CAD build for the part. Positions are in the model's coordinates, mm. A direction names the side the tool comes from. Round coordinates to 2 decimals unless told otherwise and drop trailing zeros. Loops run counter-clockwise (first coordinate to the right, second up) from the corner with the lowest first, then second, coordinate; pieces in that order, holes last. Notation, with made-up numbers: M 42.25,-19.75 L 82.25,-19.75 A25 cw 82.25,7.25 Z; hole C 34,34.5 d9. An arc over 180 degrees is marked long. Use a Markdown table: item, result. Add a question column.
(1) Band-saw the part on B-B, the plane x = 22.5. Write the cut outline in (y, z) (3 decimals), and give its area (3 significant figures).
(2) Which spindle directions (+Z, -Z, +X, -X, +Y, -Y) get a long thin tool onto all of the face, cutting with end or side? Do faces 1 (the face through (40, 2, -20.4)), 2 (the face through (23.425, 2, -35)), 3 (the face through (4, 2, -20.4)). Say none if no direction does.
(3) Band-saw the part on C-C, the plane y = 1.5. Give the number of separate pieces and of enclosed holes in the cut face, and give its area (3 significant figures).
(4) Wall check: L1, parallel to X at y = 0.65, z = -18 (3 decimals); L2, parallel to Z at x = 5, y = 2.65; L3, parallel to Z at x = 22, y = 2.8. Give the ranges that are in metal, low to high.
(5) Two-plate mould, pull along X, no slides. Class faces 4 (the face through (0, 1, -37)), 5 (the face through (30, 2, -48)), 6 (the face through (40, 1, 0)): released by +X, released by -X, zero draft, split by the parting line, or undercut.
(6) Band-saw the part on A-A, the plane x = 41. Write the cut outline in (y, z), and give its area (3 significant figures).
(7) Flat gauge pins, fed straight in: P1, Ø5, axis at x = 20, z = -11.5, coming from the -Y side; P2, Ø1.5, axis at x = 20, y = 1, coming from the -Z side. Where does each tip first touch, or does it go through?
from build123d import *

# Parameters (mm, degrees)
SKETCH1_W           = 45
SKETCH1_H           = 50
BOSS_EXTRUDE1_DEPTH = 3
SKETCH2_W           = 20
SKETCH2_H           = 3
SKETCH2_W_2         = 22
SKETCH2_W_3         = 7.5
SKETCH2_W_4         = 9
CUT_EXTRUDE1_DEPTH  = 4
SKETCH4_W           = 7.5
SKETCH4_H           = 0.1
SKETCH4_W_2         = 9
CUT_EXTRUDE2_DEPTH  = 4


with BuildPart() as part:
    # Sketch1 → Boss-Extrude1 (new body)
    with BuildSketch(Plane(origin=(0, 0, 0), x_dir=(1, 0, 0), z_dir=(0, 1, 0))):
        with Locations((22.5, 25)):
            Rectangle(SKETCH1_W, SKETCH1_H)
    extrude(amount=BOSS_EXTRUDE1_DEPTH)

    # Sketch2 → Cut-Extrude1 (cut, through all)
    with BuildSketch(Plane(origin=(0, 3, 0), x_dir=(1, 0, 0), z_dir=(0, 1, 0))):
        with Locations((20, 48.5)):
            Rectangle(SKETCH2_W, SKETCH2_H)
        with Locations((24, 1.5)):
            Rectangle(SKETCH2_W_2, SKETCH2_H)
        with Locations((3.75, 22)):
            Rectangle(SKETCH2_W_3, SKETCH2_H)
        with Locations((40.5, 22)):
            Rectangle(SKETCH2_W_4, SKETCH2_H)
        Polygon((21.050252532, 21.5), (23.949747468, 21.5), (26, 23.550252532), (26, 26.449747468), (23.949747468, 28.5), (21.050252532, 28.5), (19, 26.449747468), (19, 23.550252532), align=None)
        with BuildLine():
            Line((21.575, 31.5), (21.575, 38.25))
            ThreePointArc((21.575, 38.25), (22.5, 39.175), (23.425, 38.25))
            Line((23.425, 38.25), (23.425, 31.5))
            ThreePointArc((23.425, 31.5), (22.5, 30.575), (21.575, 31.5))
        make_face()
        with BuildLine():
            Line((23.425, 18.5), (23.425, 11.75))
            ThreePointArc((23.425, 11.75), (22.5, 10.825), (21.575, 11.75))
            Line((21.575, 11.75), (21.575, 18.5))
            ThreePointArc((21.575, 18.5), (22.5, 19.425), (23.425, 18.5))
        make_face()
    extrude(amount=-CUT_EXTRUDE1_DEPTH, mode=Mode.SUBTRACT)

    # Sketch4 → Cut-Extrude2 (cut, through all)
    with BuildSketch(Plane(origin=(0, 3, 0), x_dir=(1, 0, 0), z_dir=(0, 1, 0))):
        with Locations((3.75, 23.55)):
            Rectangle(SKETCH4_W, SKETCH4_H)
        with Locations((3.75, 20.45)):
            Rectangle(SKETCH4_W, SKETCH4_H)
        with Locations((40.5, 20.45)):
            Rectangle(SKETCH4_W_2, SKETCH4_H)
        with Locations((40.5, 23.55)):
            Rectangle(SKETCH4_W_2, SKETCH4_H)
    extrude(amount=-CUT_EXTRUDE2_DEPTH, mode=Mode.SUBTRACT)


solid = part.part
Return value:
| question | item | result |
|---|---|---|
| 1 | outline | M 0,-47 L 3,-47 L 3,-39.175 L 0,-39.175 Z; M 0,-30.575 L 3,-30.575 L 3,-28.5 L 0,-28.5 Z; M 0,-21.5 L 3,-21.5 L 3,-19.425 L 0,-19.425 Z; M 0,-10.825 L 3,-10.825 L 3,-3 L 0,-3 Z |
| 1 | area | 59.4 mm^2 |
| 2 | face 1 | +X, +Y, -Y |
| 2 | face 2 | +Y, -Y |
| 2 | face 3 | -X, +Y, -Y |
| 3 | separate pieces | 1 |
| 3 | enclosed holes | 3 |
| 3 | area | 2,000 mm^2 |
| 4 | L1 | 0 to 21.575, 23.425 to 45 |
| 4 | L2 | -50 to -23.6, -20.4 to 0 |
| 4 | L3 | -47 to -39.03, -30.72 to -28.5, -21.5 to -19.28, -10.97 to -3 |
| 5 | face 4 | released by -X |
| 5 | face 5 | undercut |
| 5 | face 6 | zero draft |
| 6 | outline | M 0,-50 L 3,-50 L 3,-23.6 L 0,-23.6 Z; M 0,-20.4 L 3,-20.4 L 3,0 L 0,0 Z |
| 6 | area | 140 mm^2 |
| 7 | P1 | y = 0 |
| 7 | P2 | z = -47 |
